Build history of the part. All positions in model axes, mm. A direction names the side the tool comes from. Give positions to 0.01 mm unless a question says otherwise; leave off trailing zeros. Order: outer loops, then holes, each group sorted by start corner. A loop starts at its lowest first (then second) coordinate and runs counter-clockwise, first axis right, second up. Notation, with made-up numbers: M 4.5,53.5 L 13.5,53.5 A21 ccw 13.5,85.5 Z; hole C 11,42.5 d11. An arc over 180 degrees is marked long. One line per item, written item: value.
Autodesk Inventor part; units mm, degrees
ref_plane "YZ Plane" through (0, 0, 0) normal (1, 0, 0) x (0, 1, 0)
ref_plane "XZ Plane" through (0, 0, 0) normal (0, 1, 0) x (-1, 0, 0)
ref_plane "XY Plane" through (0, 0, 0) normal (0, 0, 1) x (1, 0, 0)
sketch "Sketch1" plane through (0, 0, 0) normal (1, 0, 0) x (0, 1, 0)
  line L0 (0, 0) -> (50.8, 0)
  line L1 (50.8, 0) -> (50.8, -25.4)
  line L2 (50.8, -25.4) -> (0, -25.4)
  line L3 (0, -25.4) -> (0, 0)
  dimension "d0" = 50.8
  dimension "d1" = 25.4
extrude "Extrusion1" add sketch "Sketch1" along normal blind 66.675
shell "Shell1" thickness 1.5875 removed faces 2 at (0, 16.9333, -16.9333) at (66.675, 16.9333, -16.9333)
hole "Hole1" at (53.975, 12.7, 0) direction (0, 0, -1) diameter 5.1594 end through all
hole "Hole2" at (53.975, 38.1, 0) direction (0, 0, -1) diameter 5.1594 end through all
hole "Hole3" at (12.7, 38.1, 0) direction (0, 0, -1) diameter 5.1594 end through all
hole "Hole4" at (12.7, 12.7, 0) direction (0, 0, -1) diameter 5.1594 end through all
hole "Hole5" at (28.575, 38.1, -25.4) direction (0, 0, 1) diameter 5.1594 end through all
hole "Hole6" at (28.575, 12.7, -25.4) direction (0, 0, 1) diameter 5.1594 end through all
properties part number "1x2 2 625 in Beam Flywheel Mount"
1) Saw through at C-C, the plane z = -7. Write the cut outline in (x, y) (1 decimal), then the cut area to 3 significant figures.
Check values:
outline: M 0,0 L 66.7,0 L 66.7,1.6 L 0,1.6 Z; M 0,49.2 L 66.7,49.2 L 66.7,50.8 L 0,50.8 Z
area: 212 mm^2
2) Saw through at A-A, the plane x = 12.7. Write the cut outline in (y, z), then the cut area to 3 significant figures.
Check values:
outline: M 0,-25.4 L 10.12,-25.4 L 10.12,-23.81 L 1.59,-23.81 L 1.59,-1.59 L 10.12,-1.59 L 10.12,0 L 0,0 Z; M 15.28,-25.4 L 35.52,-25.4 L 35.52,-23.81 L 15.28,-23.81 Z; M 15.28,-1.59 L 35.52,-1.59 L 35.52,0 L 15.28,0 Z; M 40.68,-25.4 L 50.8,-25.4 L 50.8,0 L 40.68,0 L 40.68,-1.59 L 49.21,-1.59 L 49.21,-23.81 L 40.68,-23.81 Z
area: 199 mm^2
3) Mould opens along Z. For faces 3 (the face through (33, 25, -1.588)), 4 (the face through (33, 25, 0)), 5 (the face through (33, 26, -25.4)), 6 (the face through (52.23, 40, -24.62)) say: released by +Z, released by -Z, zero draft, split by the parting line, or undercut.
Check values:
face 3: undercut
face 4: released by +Z
face 5: released by -Z
face 6: zero draft
4) Tool access for faces 1 (the face through (33, 1.588, -13)), 2 (the face through (12.587, 40.677, -0.805)): list every direction of +Z, -Z, +X, -X, +Y, -Y with a clear straight run to the whole face (end or side of a thin tool).
Check values:
face 1: +X, -X
face 2: +Z, -Z
5) Saw through at D-D, the plane y = 46. Write the cut outline in (x, z) (1 decimal).
Check values:
outline: M 0,-25.4 L 66.7,-25.4 L 66.7,-23.8 L 0,-23.8 Z; M 0,-1.6 L 66.7,-1.6 L 66.7,0 L 0,0 Z
6) Saw through at B-B, the plane y = 12.7. Give the number of separate pieces and of enclosed holes in the cut face, then the cut area to 3 significant figures.
Check values:
separate pieces: 8
enclosed holes: 0
area: 163 mm^2
7) Drill centre lines: probe 1 along Y at (x, z) = (12.7, -24.35); probe 2 along X at (y, z) = (12.7, -24.6) (3 decimals); probe 3 along Y at (x, z) = (45.5, -23). Where is each one in solid material? Low to high. Write a range as from..to.
Check values:
probe 1: 0..10.12, 15.28..35.52, 40.68..50.8
probe 2: 0..10.12, 15.28..25.995, 31.155..51.395, 56.555..66.675
probe 3: 0..1.59, 49.21..50.8
